Model file for the job. Use its own axes, mm. Face numbers are marked on the shaded views. Round coordinates to 2 decimals unless told otherwise and drop trailing zeros. Loops run counter-clockwise (first coordinate to the right, second up) from the corner with the lowest first, then second, coordinate; pieces in that order, holes last. Notation, with made-up numbers: (85.5, 6.25) -> (105.5, 6.25) arc R6 ccw to (105.5, 13.25) -> close; hole circle Ø4 at (32, -4). An arc over 180 degrees is marked (long way). Use a Markdown table: item, result. Add a question column.
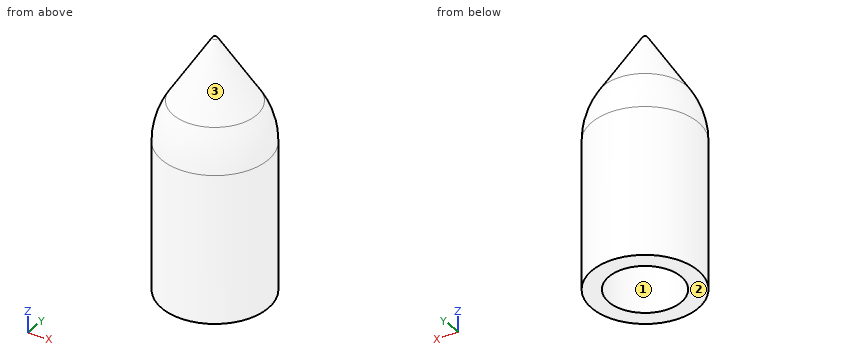
Autodesk Fusion 360 part; units mm, degrees
sketch "Schizzo2" plane through (0, 0, 0) normal (0, 1, 0) x (1, 0, 0)
  line L0 (6.25, 0) -> (6.25, -17.4188)
  line L1 (0.2968, -29.5251) -> (4.882, -22.1888)
  line L2 (0, -26.2264) -> (0, -29.6896)
  arc A0 (4.882, -22.1888) -> (6.25, -17.4188) centre (-2.75, -17.4188) ccw
  line L3 (0.9375, -28.5) -> (0, -28.5) construction
  arc A1 (0, -29.6896) -> (0.2968, -29.5251) centre (0, -29.3396) ccw
  line L4 (0, -26.2264) -> (3.186, -21.1288)
  arc A2 (3.186, -21.1288) -> (4.25, -17.4188) centre (-2.75, -17.4188) ccw
  line L5 (4.25, 0) -> (4.25, -17.4188)
  line L6 (6.25, 0) -> (4.25, 0)
  dimension "d9" = 6.25
  dimension "d24" = 9
  dimension "d25" = 0.35
revolve "Rivoluzione6" add sketch "Schizzo2" angle 360 about axis through (0, 0, 26.2264) along (0, 0, 1)
revolve "Rivoluzione5" [suppressed]
revolve "Rivoluzione3" [suppressed]
ref_plane "Piano di lavoro1" through (0, -3, 0) normal (0, 1, 0) x (0, 0, 1)
revolve "Rivoluzione4" [suppressed]
revolve "Rivoluzione2" [suppressed]
sketch "Schizzo3" plane through (0, 0, 0) normal (0, 1, 0) x (1, 0, 0)
  line L0 (0, 1) -> (0, -23)
revolve "Rivoluzione1" [suppressed]
equation "d9 = ( 12.5 / 2 ) * 1 mm"
1) Pull direction X, two halves, no side cores. Call the marked faces 1, 2 and 3: +X half, -X half, draft (parallel to the pull), parting line (faces both ways), or undercut.
2) Cut at A-A on z = 7.25. Write the cut outline in (x, y), and give its area (3 significant figures).
3) Pin check, flat tips, straight feed: pin 1 Ø1 at (x, y) = (0, 1.5) entering from +Z; pin 2 Ø3 at (x, y) = (1.5, 0) entering from -Z; pin 3 Ø1.5 at (y, z) = (1, 7.5) entering from +X (3 decimals). Stop position of each tip, or through.
4) Wall check: probe 1 along Y at (x, z) = (0, 8); probe 2 along X at (y, z) = (-2.25, 12); probe 3 along X at (y, z) = (-0.5, 21). Give the ranges that are in metal, low to high. Write a range as from..to.
Established:
| question | item | result |
|---|---|---|
| 1 | face 1 | undercut |
| 1 | face 2 | draft |
| 1 | face 3 | parting line |
| 2 | outline | circle Ø12.5 at (0, 0); hole circle Ø8.5 at (0, 0) |
| 2 | area | 66.0 mm^2 |
| 3 | pin 1 | stops at z = 28.4 |
| 3 | pin 2 | stops at z = 21.43 |
| 3 | pin 3 | stops at x = 6.245 |
| 4 | probe 1 | y = -6.25..-4.25, 4.25..6.25 |
| 4 | probe 2 | x = -5.83..-3.61, 3.61..5.83 |
| 4 | probe 3 | x = -5.48..-3.23, 3.23..5.48 |
